Can you work these out from the model? Positions are in its coordinate system, mm. A direction names the side the tool comes from. Coordinates: 2 decimals unless noted, no trailing zeros. Order: outer loops, then holes, each group sorted by start corner. A loop starts at its lowest first (then second) coordinate and runs counter-clockwise, first axis right, second up. Notation, with made-up numbers: (-11, -33.75) -> (12, -33.75) arc R21 ccw to (12, 3.25) -> close; hole circle Ø1 at (-29.75, -40). An arc over 180 degrees is marked (long way). Write item = value, one per line. Start each with the question number.
from build123d import *

# Parameters (mm, degrees)
SKETCH1_W                 = 55
SKETCH1_H                 = 55
BOSS_EXTRUDE1_DEPTH       = 5
SKETCH2_W                 = 5
SKETCH2_H                 = 55
BOSS_EXTRUDE2_DEPTH       = 100
CUT_EXTRUDE1_REACH        = 57
SKETCH3_R                 = 5
SKETCH3_R_2               = 1.5
SKETCH3_R_3               = 11
CUT_EXTRUDE2_REACH        = 7
SKETCH4_R                 = 4
F_4_48_TAPPED_HOLE1_D     = 2.3749
F_4_48_TAPPED_HOLE1_DEPTH = 3.5
F_4_48_TAPPED_HOLE1_TIP   = 0.713491942


with BuildPart() as part:
    # Sketch1 → Boss-Extrude1 (new body)
    with BuildSketch(Plane.XY):
        Rectangle(SKETCH1_W, SKETCH1_H)
    extrude(amount=BOSS_EXTRUDE1_DEPTH)

    # Sketch2 → Boss-Extrude2 (add)
    with BuildSketch(Plane.XY.offset(5)):
        with Locations((25, 0)):
            Rectangle(SKETCH2_W, SKETCH2_H)
    extrude(amount=BOSS_EXTRUDE2_DEPTH)

    # Sketch3 → Cut-Extrude1 (cut, up to next)
    with BuildSketch(Plane(origin=(27.5, 0, 0), x_dir=(0, 0, -1), z_dir=(1, 0, 0)), mode=Mode.PRIVATE) as cut_extrude1_sk1:
        with Locations((-95, 0)):
            Circle(SKETCH3_R)
    cut_extrude1_tool1 = extrude(cut_extrude1_sk1.sketch, amount=-CUT_EXTRUDE1_REACH, mode=Mode.PRIVATE) & part.part
    add(cut_extrude1_tool1.solids().sort_by_distance((27.5, 0, 95))[0], mode=Mode.SUBTRACT)
    # Sketch3 → Cut-Extrude1 (cut, up to next)
    with BuildSketch(Plane(origin=(27.5, 0, 0), x_dir=(0, 0, -1), z_dir=(1, 0, 0)), mode=Mode.PRIVATE) as cut_extrude1_sk2:
        with Locations((-95, 25)):
            Circle(SKETCH3_R_2)
    cut_extrude1_tool2 = extrude(cut_extrude1_sk2.sketch, amount=-CUT_EXTRUDE1_REACH, mode=Mode.PRIVATE) & part.part
    add(cut_extrude1_tool2.solids().sort_by_distance((27.5, 25, 95))[0], mode=Mode.SUBTRACT)
    # Sketch3 → Cut-Extrude1 (cut, up to next)
    with BuildSketch(Plane(origin=(27.5, 0, 0), x_dir=(0, 0, -1), z_dir=(1, 0, 0)), mode=Mode.PRIVATE) as cut_extrude1_sk3:
        with Locations((-95, -25)):
            Circle(SKETCH3_R_2)
    cut_extrude1_tool3 = extrude(cut_extrude1_sk3.sketch, amount=-CUT_EXTRUDE1_REACH, mode=Mode.PRIVATE) & part.part
    add(cut_extrude1_tool3.solids().sort_by_distance((27.5, -25, 95))[0], mode=Mode.SUBTRACT)
    # Sketch3 → Cut-Extrude1 (cut, up to next)
    with BuildSketch(Plane(origin=(27.5, 0, 0), x_dir=(0, 0, -1), z_dir=(1, 0, 0)), mode=Mode.PRIVATE) as cut_extrude1_sk4:
        with Locations((-77.5, 0)):
            Circle(SKETCH3_R_3)
    cut_extrude1_tool4 = extrude(cut_extrude1_sk4.sketch, amount=-CUT_EXTRUDE1_REACH, mode=Mode.PRIVATE) & part.part
    add(cut_extrude1_tool4.solids().sort_by_distance((27.5, 0, 77.5))[0], mode=Mode.SUBTRACT)

    # Sketch4 → Cut-Extrude2 (cut, up to next)
    with BuildSketch(Plane.XY.offset(5), mode=Mode.PRIVATE) as cut_extrude2_sk1:
        Circle(SKETCH4_R)
    cut_extrude2_tool1 = extrude(cut_extrude2_sk1.sketch, amount=-CUT_EXTRUDE2_REACH, mode=Mode.PRIVATE) & part.part
    add(cut_extrude2_tool1.solids().sort_by_distance((0, 0, 5))[0], mode=Mode.SUBTRACT)

    # #4-48 Tapped Hole1
    with Locations(Plane.XY.offset(5)):
        with Locations((-17.3, 15.5), (-17.3, -15.5)):
            Hole(F_4_48_TAPPED_HOLE1_D / 2, depth=F_4_48_TAPPED_HOLE1_DEPTH)
            with Locations((0, 0, -(F_4_48_TAPPED_HOLE1_DEPTH + F_4_48_TAPPED_HOLE1_TIP / 2))):  # 118° drill point
                Cone(0, F_4_48_TAPPED_HOLE1_D / 2, F_4_48_TAPPED_HOLE1_TIP, mode=Mode.SUBTRACT)


solid = part.part
(1) For faces 1 (the face through (-8, 0, 5)), 2 (the face through (-18.4, -15.95, 3.23)), 3 (the face through (25.035, 26.265, 94.194)), which set-ups out of +Z, -Z, +X, -X, +Y, -Y let a thin tool reach every point of the face, with its end or its side?
(2) Imagine slicing it at B-B (z = 95). Write out the boundary of the cut face in (x, y), plus the area to 3 significant figures.
(3) For P1, Ø4, axis at x = -17.3, y = 15.5, coming from the +Z side; P2, Ø2.5, axis at y = -25, z = 95, coming from the -X side; P3, Ø16.5, axis at y = 3.5, z = 73, coming from the -X side, each with a flat end and sliding along its axis, tell me the tip position at first contact or that it passes through.
(4) Thinking about a two-plate mould opening in X: for faces 4 (the face through (22.5, 0, 54)), 5 (the face through (25, 0, 105)), 6 (the face through (-18.4, 15.05, 3.23)), 7 (the face through (27.5, 0, 52)), which applies, +X half, -X half, draft (parallel to the pull), parting line (faces both ways), or undercut?
(5) Imagine slicing it at C-C (y = 0). Write out the boundary of the cut face in (x, z).
(6) Imagine slicing it at D-D (y = -22). Write out the boundary of the cut face in (x, z), plus the area to 3 significant figures.
(7) Imagine slicing it at A-A (y = 25). Write out the boundary of the cut face in (x, z), plus the area to 3 significant figures.
(8) If I drill on L1, parallel to Y at x = -17.3, z = 3.9; L2, parallel to Y at x = 25.7, z = 95; L3, parallel to Y at x = -17, z = 3, over which ranges is the centre line in solid material (lowest first)? Write a range as from..to.
Result set:
q1.face_1 = +Z, -X, +Y, -Y
q1.face_2 = +Z
q1.face_3 = +X, -X
q2.outline = (22.5, -27.5) -> (27.5, -27.5) -> (27.5, -26.5) -> (22.5, -26.5) -> close; (22.5, -23.5) -> (27.5, -23.5) -> (27.5, -5) -> (22.5, -5) -> close; (22.5, 5) -> (27.5, 5) -> (27.5, 23.5) -> (22.5, 23.5) -> close; (22.5, 26.5) -> (27.5, 26.5) -> (27.5, 27.5) -> (22.5, 27.5) -> close
q2.area = 195 mm2
q3.P1 = 5
q3.P2 = through
q3.P3 = 22.5
q4.face_4 = -X half
q4.face_5 = draft
q4.face_6 = undercut
q4.face_7 = +X half
q5.outline = (-27.5, 0) -> (-4, 0) -> (-4, 5) -> (-27.5, 5) -> close; (4, 0) -> (27.5, 0) -> (27.5, 66.5) -> (22.5, 66.5) -> (22.5, 5) -> (4, 5) -> close; (22.5, 88.5) -> (27.5, 88.5) -> (27.5, 90) -> (22.5, 90) -> close; (22.5, 100) -> (27.5, 100) -> (27.5, 105) -> (22.5, 105) -> close
q6.outline = (-27.5, 0) -> (27.5, 0) -> (27.5, 105) -> (22.5, 105) -> (22.5, 5) -> (-27.5, 5) -> close
q6.area = 775 mm2
q7.outline = (-27.5, 0) -> (27.5, 0) -> (27.5, 93.5) -> (22.5, 93.5) -> (22.5, 5) -> (-27.5, 5) -> close; (22.5, 96.5) -> (27.5, 96.5) -> (27.5, 105) -> (22.5, 105) -> close
q7.area = 760 mm2
q8.L1 = -27.5..-16.69, -14.31..14.31, 16.69..27.5
q8.L2 = -27.5..-26.5, -23.5..-5, 5..23.5, 26.5..27.5
q8.L3 = -27.5..-16.65, -14.35..14.35, 16.65..27.5
